Autodesk Inventor part; units mm, degrees
ref_plane "YZ Plane" through (0, 0, 0) normal (1, 0, 0) x (0, 1, 0)
ref_plane "XZ Plane" through (0, 0, 0) normal (0, 1, 0) x (-1, 0, 0)
ref_plane "XY Plane" through (0, 0, 0) normal (0, 0, 1) x (1, 0, 0)
sketch "Sketch1" plane through (0, 0, 0) normal (0, 1, 0) x (-1, 0, 0)
  line L0 (40, 43) -> (40, -43)
  line L1 (40, -43) -> (-40, -43)
  line L2 (-40, -43) -> (-40, 43)
  line L3 (-40, 43) -> (40, 43)
  line L4 (40, 43) -> (-40, -43) construction
  line L5 (40, -43) -> (-40, 43) construction
  point P0 (0, 0)
  dimension "d0" = 86
  dimension "d1" = 80
extrude "Extrusion1" add sketch "Sketch1" along normal blind 5
sketch "Sketch2" plane through (40, 0, -43) normal (0, 0, -1) x (-1, 0, 0)
  line L0 (0, 0) -> (80, 0)
  line L1 (80, 0) -> (80, 5)
  line L2 (0, 5) -> (80, 5)
  line L3 (0, 0) -> (0, 5)
  circle A0 centre (40.1562, 2.5) radius 1.5
  dimension "d4" = 3
extrude "Extrusion2" cut sketch "Sketch2" against normal blind 6 contours A0
sketch "Sketch3" plane through (-40, 0, 43) normal (0, 0, 1) x (1, 0, 0)
  line L0 (0, 0) -> (80, 0)
  line L1 (80, 0) -> (80, 5)
  line L2 (0, 5) -> (80, 5)
  line L3 (0, 0) -> (0, 5)
  circle A0 centre (40, 2.5) radius 2.5
  dimension "d7" = 5
extrude "Extrusion3" add sketch "Sketch3" along normal blind 1 contours A0
sketch "Sketch4" plane through (0, 2.5, 44) normal (0, 0, 1) x (1, 0, 0)
  circle A0 centre (0, 0) radius 1.5
  dimension "d10" = 3
extrude "Extrusion4" add sketch "Sketch4" along normal blind 4
properties part number "brush"
Geometry: final body of the model. Coordinates: model frame, mm. A direction names the side the tool comes from. Coordinates: 2 decimals unless noted, no trailing zeros. Order: outer loops, then holes, each group sorted by start corner. A loop starts at its lowest first (then second) coordinate and runs counter-clockwise, first axis right, second up. Notation, with made-up numbers: (79.25, 72) -> (127.25, 72) arc R21 cw to (127.25, 88) -> close; hole circle Ø4 at (15.5, -30). An arc over 180 degrees is marked (long way). Write each question's results on one line, items separated by ' | '. Start each with the question number.
1) First-contact query: pin 1 (0.9 mm diameter, centred on x = 0.5, y = 2.5, fed in from -Z); pin 2 (1.5 mm diameter, centred on x = 15, y = 1, fed in from +Z). Flat tips, straight axial feed; report the tip coordinate or a pass-through.
2) Mould query, pull axis X, two halves, no side actions, for faces 4 (the flat face through (40, 2, -1)), 5 (the flat face through (0, 3, -37)), 6 (the flat face through (-40, 2, 1)). Classes: released by +X, released by -X, zero draft, split by the parting line, or undercut.
3) Cut plane B-B, the plane x = 23. Output: boundary loops of the cut face in (y, z).
4) Cut plane A-A, the plane y = 2.5. Output: boundary loops of the cut face in (x, z).
5) Set-up query: faces 1 (the cylindrical face through (0, 1, 46)), 2 (the flat face through (1, 0, 1)), 3 (the cylindrical face through (0.169, 1.036, -40.042)). Return all of +Z, -Z, +X, -X, +Y, -Y with unobstructed straight access to the full face (end or side cutting, diameter ignored); none if empty.
6) Material intervals for line 1 along Z through (x, y) = (31, 1.65), sorted ascending.
Checks:
1) pin 1: z = -37 | pin 2: z = 43
2) face 4: released by +X | face 5: undercut | face 6: released by -X
3) outline: (0, -43) -> (5, -43) -> (5, 43) -> (0, 43) -> close
4) outline: (-40, -43) -> (-1.66, -43) -> (-1.66, -37) -> (1.34, -37) -> (1.34, -43) -> (40, -43) -> (40, 43) -> (2.5, 43) -> (2.5, 44) -> (1.5, 44) -> (1.5, 48) -> (-1.5, 48) -> (-1.5, 44) -> (-2.5, 44) -> (-2.5, 43) -> (-40, 43) -> close
5) face 1: +Z | face 2: +Z, -Z, +X, -X, -Y | face 3: -Z
6) line 1: -43 to 43
